Solid Edge part; units mm, degrees
sketch "Sketch1" plane through (0, 0, 0) normal (0, 0, 1) x (1, 0, 0)
  line L0 (-1.3856, 2.4) -> (1.3856, 2.4)
  line L1 (1.3856, 2.4) -> (2.7713, 0)
  line L2 (2.7713, 0) -> (1.3856, -2.4)
  line L3 (1.3856, -2.4) -> (-1.3856, -2.4)
  line L4 (-1.3856, -2.4) -> (-2.7713, 0)
  line L5 (-2.7713, 0) -> (-1.3856, 2.4)
extrude "Protrusion1" add sketch "Sketch1" along normal blind 0.5
sketch "Sketch2" plane through (0, 0, 0.5) normal (0, 0, 1) x (1, 0, 0)
  circle A0 centre (0, 0) radius 2.1
extrude "Ausprägung_2" add sketch "Sketch2" along normal blind 9.5
hole "Bohrung_1" at (0, 0, 10) direction (0, 0, -1) diameter 3 depth 5
chamfer "Fase_1" distance 0.2 angle 45 1 edges at (0, 1.5, 10)
Geometry: final body of the model. Coordinates: model frame, mm. A direction names the side the tool comes from. Round coordinates to 2 decimals unless told otherwise and drop trailing zeros. Write each loop counter-clockwise with the first axis right and the second up, starting at its lowest first coordinate (ties: lowest second). Pieces come first, ordered by that corner, then holes. Notation, with made-up numbers: M 83,36 L 89,36 A28 cw 89,73 Z; hole C 87.25,-39.75 d10. An arc over 180 degrees is marked long. Write item = value, one per line.
Item 1: Section query B-B on x = 0. Return loops of the section in (y, z).
Findings:
outline = M -2.4,0 L 2.4,0 L 2.4,0.5 L 2.1,0.5 L 2.1,10 L 1.7,10 L 1.5,9.8 L 1.5,5 L -1.5,5 L -1.5,9.8 L -1.7,10 L -2.1,10 L -2.1,0.5 L -2.4,0.5 Z
Item 2: Material intervals for line 1 along Y through (x, z) = (0, 8.25); line 2 along Y through (x, z) = (-0.05, 1); line 3 along Z through (x, y) = (0.15, 1.45), sorted ascending. Write a range as [from, to].
Findings:
line_1 = [-2.1, -1.5], [1.5, 2.1]
line_2 = [-2.1, 2.1]
line_3 = [0, 5]
Item 3: Section query C-C on y = -1.85. Return loops of the section in (x, z), then the cut area to 3 significant figures.
Findings:
outline = M -1.7,0 L 1.7,0 L 1.7,0.5 L 0.99,0.5 L 0.99,10 L -0.99,10 L -0.99,0.5 L -1.7,0.5 Z
area = 20.6 mm^2
Item 4: Access query for faces 4 (the face through (-2.069, -1.217, 0.246)), 5 (the face through (2.003, -0.631, 5.184)). Directions: +Z, -Z, +X, -X, +Y, -Y. A direction counts if a zero-diameter tool reaches every point of the face in a straight line with its end or side. Return the directions, or none.
Findings:
face_4 = +Z, -Z, -X, -Y
face_5 = +Z
Item 5: Pin query (flat end, axial travel): P1, Ø1.5, axis at y = 0.5, z = 8.5, coming from the +X side; P2, Ø0.9, axis at x = -0.5, y = 0.5, coming from the +Z side; P3, Ø3, axis at x = 2, z = 3, coming from the +Y side. Return the tip coordinate at first contact, or that it passes through.
Findings:
P1 = 2.1
P2 = 5
P3 = 2.04
Item 6: Section query D-D on z = 4.25. Return loops of the section in (x, y).
Findings:
outline = C 0,0 d4.2
Item 7: Section query A-A on z = 6.75. Return loops of the section in (x, y).
Findings:
outline = C 0,0 d4.2; hole C 0,0 d3
Item 8: Pull-direction query (X, two-part tool) for faces 1 (the face through (0, 0, 0)), 2 (the face through (0, 0, 5)), 3 (the face through (2.09, -1.18, 0.25)); classes: pulls with the +X half, pulls with the -X half, needs draft (parallel to the pull), parting line crosses it, or undercut.
Findings:
face_1 = needs draft
face_2 = undercut
face_3 = pulls with the +X half
